from build123d import *

# Parameters (mm, degrees)
SKETCH1_W                               = 47.625
SKETCH1_H                               = 33.3502
BOSS_EXTRUDE1_DEPTH                     = 44.45
SKETCH2_W                               = 47.625
SKETCH2_H                               = 20.6502
CUT_EXTRUDE1_DEPTH                      = 34.925
CUT_EXTRUDE2_DEPTH                      = 1
CUT_EXTRUDE2_DEPTH_BACK                 = 34.3502
CBORE_FOR_M8_HEX_HEAD_BOLT1_D           = 9
CBORE_FOR_M8_HEX_HEAD_BOLT1_DEPTH       = 13.298127214
CBORE_FOR_M8_HEX_HEAD_BOLT1_CBORE_D     = 16
CBORE_FOR_M8_HEX_HEAD_BOLT1_CBORE_DEPTH = 5.3
CBORE_FOR_M8_HEX_HEAD_BOLT1_TIP         = 2.703872786
FILLET3_R                               = 6.35
F_3_8_0_375_DIAMETER_HOLE1_D            = 9.525


with BuildPart() as part:
    # Sketch1 → Boss-Extrude1 (new body)
    with BuildSketch(Plane(origin=(0, 0, 0), x_dir=(1, 0, 0), z_dir=(0, 1, 0))):
        Rectangle(SKETCH1_W, SKETCH1_H)
    extrude(amount=BOSS_EXTRUDE1_DEPTH)

    # Sketch2 → Cut-Extrude1 (cut)
    with BuildSketch(Plane(origin=(0, 44.45, 0), x_dir=(1, 0, 0), z_dir=(0, 1, 0))):
        Rectangle(SKETCH2_W, SKETCH2_H)
    extrude(amount=-CUT_EXTRUDE1_DEPTH, mode=Mode.SUBTRACT)

    # Sketch3 → Cut-Extrude2 (cut, two sides)
    with BuildSketch(Plane(origin=(0, 0, -16.6751), x_dir=(-1, 0, 0), z_dir=(0, 0, -1))) as cut_extrude2_sk:
        Polygon((23.8125, 44.45), (9.525, 44.45), (23.8125, 9.525), align=None)
        Polygon((-23.8125, 9.525), (-9.525, 44.45), (-23.8125, 44.45), align=None)
    extrude(amount=CUT_EXTRUDE2_DEPTH, mode=Mode.SUBTRACT)
    extrude(cut_extrude2_sk.sketch, amount=-CUT_EXTRUDE2_DEPTH_BACK, mode=Mode.SUBTRACT)

    # CBORE for M8 Hex Head Bolt1
    with Locations(Plane(origin=(0, 9.525, 0), x_dir=(1, 0, 0), z_dir=(0, 1, 0))):
        with Locations((-12.7, 0), (12.7, 0)):
            CounterBoreHole(CBORE_FOR_M8_HEX_HEAD_BOLT1_D / 2, CBORE_FOR_M8_HEX_HEAD_BOLT1_CBORE_D / 2, CBORE_FOR_M8_HEX_HEAD_BOLT1_CBORE_DEPTH, depth=CBORE_FOR_M8_HEX_HEAD_BOLT1_DEPTH)
            with Locations((0, 0, -(CBORE_FOR_M8_HEX_HEAD_BOLT1_DEPTH + CBORE_FOR_M8_HEX_HEAD_BOLT1_TIP / 2))):  # 118° drill point
                Cone(0, CBORE_FOR_M8_HEX_HEAD_BOLT1_D / 2, CBORE_FOR_M8_HEX_HEAD_BOLT1_TIP, mode=Mode.SUBTRACT)

    # Fillet3
    fillet3_edges = [part.edges().sort_by_distance(p)[0] for p in [
        (9.525, 44.45, 13.5001),
        (-9.525, 44.45, 13.5001),
        (9.525, 44.45, -13.5001),
        (-9.525, 44.45, -13.5001),
    ]]
    fillet(fillet3_edges, radius=FILLET3_R)

    # 3/8 (0.375) Diameter Hole1 (through all)
    with Locations(Plane.XY.offset(16.6751)):
        with Locations((0, 25.161662577)):
            Hole(F_3_8_0_375_DIAMETER_HOLE1_D / 2)


solid = part.part
Work out the finished part from the listing and answer in its coordinate system (mm). A direction names the side the tool comes from. Round coordinates to 2 decimals unless told otherwise and drop trailing zeros. Order: outer loops, then holes, each group sorted by start corner. A loop starts at its lowest first (then second) coordinate and runs counter-clockwise, first axis right, second up. Notation, with made-up numbers: M -9.5,16 L 5.5,16 A24 ccw 5.5,30 Z; hole C 52.5,28 d1. An arc over 180 degrees is marked long. Put each result on its own line as item: value. Start each with the question number.
Q1. Flat-ended cylindrical pins translate along their axes: pin 1 (12 mm diameter, centred on y = 32.5, z = -5, fed in from +X); pin 2 (5 mm diameter, centred on x = -14.5, z = 4, fed in from +Y) (3 decimals); pin 3 (5 mm diameter, centred on y = 22.5, z = 11.5, fed in from -X). Find the tip coordinate at first contact, or state that the pin passes through.
Q2. Section A-A, the plane x = 0 is taken. Write down the section's boundary in (y, z) (3 decimals).
Q3. For a pull along X with two mould halves and no side action, classify faces 1 (the flat face through (5, 23, -10.325)), 2 (the cylindrical face through (8.845, 43.343, -13.456)), 3 (the flat face through (-9, 4.225, 3)) as pulls with the +X half, pulls with the -X half, needs draft (parallel to the pull), parting line crosses it, or undercut.
Q4. Section B-B, the plane y = 35.5 is taken. Write down the section's boundary in (x, z), and give its area (3 significant figures).
Q5. A tool of negligible diameter and unlimited length cuts with its end or side. For faces 4 (the flat face through (0, 0, 0)), 5 (the flat face through (16.1, 4.225, 3.4)), 6 (the flat face through (0, 9.525, 0)), from which of +Z, -Z, +X, -X, +Y, -Y can it reach the whole face along a straight path? Write none if from no direction.
Q6. Section D-D, the plane y = 27 is taken. Write down the section's boundary in (x, z), and give its area (3 significant figures).
Q7. Section C-C, the plane x = 12.7 is taken. Write down the section's boundary in (y, z) (3 decimals), and give its area (3 significant figures).
Q8. Straight lines are drawn through the part: L1, parallel to Z at x = 8.5, y = 19.5; L2, parallel to Z at x = 12.7, y = 6.65; L3, parallel to X at y = 6, z = -1.5. For each, find the intervals that lie inside material, in ascending order. Write a range as [from, to].
Findings below:
1. pin 1: stops at x = 15.54
1. pin 2: stops at y = 4.225
1. pin 3: stops at x = -19.53
2. outline: M 0,-16.675 L 20.399,-16.675 L 20.399,-10.325 L 9.525,-10.325 L 9.525,10.325 L 20.399,10.325 L 20.399,16.675 L 0,16.675 Z; M 29.924,-16.675 L 44.45,-16.675 L 44.45,-10.325 L 29.924,-10.325 Z; M 29.924,10.325 L 44.45,10.325 L 44.45,16.675 L 29.924,16.675 Z
3. face 1: needs draft
3. face 2: pulls with the +X half
3. face 3: undercut
4. outline: M -13.19,-16.68 L 13.19,-16.68 L 13.19,-10.33 L -13.19,-10.33 Z; M -13.19,10.33 L 13.19,10.33 L 13.19,16.68 L -13.19,16.68 Z
4. area: 335 mm^2
5. face 4: +Z, -Z, +X, -X, -Y
5. face 5: +Y
5. face 6: +X, -X, +Y
6. outline: M -16.66,-16.68 L -4.39,-16.68 L -4.39,-10.33 L -16.66,-10.33 Z; M -16.66,10.33 L -4.39,10.33 L -4.39,16.68 L -16.66,16.68 Z; M 4.39,-16.68 L 16.66,-16.68 L 16.66,-10.33 L 4.39,-10.33 Z; M 4.39,10.33 L 16.66,10.33 L 16.66,16.68 L 4.39,16.68 Z
6. area: 312 mm^2
7. outline: M 0,-16.675 L 36.689,-16.675 L 36.689,-10.325 L 9.525,-10.325 L 9.525,-8 L 4.225,-8 L 4.225,-4.5 L 0,-4.5 Z; M 0,4.5 L 4.225,4.5 L 4.225,8 L 9.525,8 L 9.525,10.325 L 36.689,10.325 L 36.689,16.675 L 0,16.675 Z
7. area: 540 mm^2
8. L1: z = [-16.68, -10.33], [10.33, 16.68]
8. L2: z = [-16.68, -8], [8, 16.68]
8. L3: x = [-23.81, -20.56], [-4.84, 4.84], [20.56, 23.81]
